The listing builds one solid part. Answer for the finished solid, in the listing's coordinates (mm). A direction names the side the tool comes from. Round coordinates to 2 decimals unless told otherwise and drop trailing zeros. Write each loop counter-clockwise with the first axis right and the second up, starting at its lowest first coordinate (ties: lowest second). Pieces come first, ordered by that corner, then holes.
Item 1: Find section B-B on x = 0. Give the vertices of the cut face in (y, z) (3 decimals), then the cut area to 3 significant figures.
Item 2: For a pull along Y with two mould halves and no side action, classify faces 1 (the face through (0.833, -2, 6)), 2 (the face through (0.2, 12.7, 11.1)), 3 (the face through (9.5, 0, 11)) as +Y half, -Y half, draft (parallel to the pull), parting line (faces both ways), or undercut.
Item 3: Find the intervals of material crossed by probe 1 along X at (y, z) = (-0.25, 9); probe 2 along X at (y, z) = (3, 5.5); probe 3 along X at (y, z) = (-2.75, 10), in increasing order.
Item 4: Find section A-A on z = 10.5. Give the vertices of the cut face in (x, y), then the cut area to 3 significant figures.
Item 5: Find section C-C on y = 8.75. Give the vertices of the cut face in (x, z) (3 decimals).
Item 6: Each of these flat-tipped pins is pushed along its axis until it touches: pin 1 (1.8 mm diameter, centred on x = -0.5, z = 9, fed in from -Y); pin 2 (2.5 mm diameter, centred on x = -2, z = 9, fed in from +Y); pin 3 (2 mm diameter, centred on y = -3, z = 3.5, fed in from -X); pin 4 (4 mm diameter, centred on x = -5.5, z = 9, fed in from -Y). Where does it stop, or does it pass through?
Item 7: A tool of negligible diameter and unlimited length cuts with its end or side. For faces 4 (the face through (1, -10, 9.525)), 5 (the face through (0, 10, 9.525)), 6 (the face through (2, -1.13, 6)), 7 (the face through (-2, 3, 12.7)), from which of +Z, -Z, +X, -X, +Y, -Y can it reach the whole face along a straight path? Write none if from no direction.
Item 8: Find section D-D on x = -6.5. Give the vertices of the cut face in (y, z) (3 decimals).
```python
from build123d import *

# Parameters (mm, degrees)
F0_R     = 9.4996
F1_DEPTH = 9.525
F2_R     = 12.7
F2_R_2   = 9.4996
F3_DEPTH = 3.175
F5_DEPTH = 25.4
F7_DEPTH = 25.4
F9_DEPTH = 25.4


with BuildPart() as f1:
    # F0 (on Top) → F1 (new body)
    with BuildSketch(Plane.XY):
        Circle(F0_R)
    extrude(amount=F1_DEPTH)

    # F2 (on face) → F3 (join)
    with BuildSketch(Plane.XY.offset(9.525)):
        Circle(F2_R)
        Circle(F2_R_2, mode=Mode.SUBTRACT)
        Circle(F2_R_2)
    extrude(amount=F3_DEPTH)

    # F4 (on face) → F5 (cut)
    with BuildSketch(Plane.XY.offset(12.7)):
        with BuildLine():
            ThreePointArc((-9.4996, 8.428974), (-12.7, 0), (-9.4996, -8.428974))
            Line((-9.4996, -8.428974), (-9.4996, 8.428974))
        make_face()
        with BuildLine():
            Line((9.4996, 8.428974), (9.4996, -8.428974))
            ThreePointArc((9.4996, -8.428974), (11.872972, -4.508053), (12.7, 0))
            ThreePointArc((12.7, 0), (11.872972, 4.508053), (9.4996, 8.428974))
        make_face()
    extrude(amount=-F5_DEPTH, mode=Mode.SUBTRACT)

    # F6 (on face) → F7 (cut)
    with BuildSketch(Plane.XY.offset(12.7)):
        with BuildLine():
            ThreePointArc((2.8575, -3.421372), (4.037881, -1.888546), (4.4577, 0))
            ThreePointArc((4.4577, 0), (4.037881, 1.888546), (2.8575, 3.421372))
            Line((2.8575, 3.421372), (2.8575, -3.421372))
        make_face()
        with BuildLine():
            Line((-2.8575, -3.421372), (-2.8575, 3.421372))
            ThreePointArc((-2.8575, 3.421372), (-4.4577, 0), (-2.8575, -3.421372))
        make_face()
    extrude(amount=-F7_DEPTH, mode=Mode.SUBTRACT)

    # F8 (on face) → F9 (cut)
    with BuildSketch(Plane(origin=(0, 0, 0), x_dir=(1, 0, 0), z_dir=(0, 0, -1))):
        Polygon((-2.8575, 2.16922), (-2.8575, -2.392801), (-0.969418, -2.392801), (-0.969418, -3.421372), (1.220574, -3.421372), (1.220574, -2.392801), (2.8575, -2.392801), (2.8575, 1.130344), (0.832597, 1.130344), (0.832597, 3.162927), (-0.79347, 3.162927), (-0.79347, 2.16922), align=None)
    extrude(amount=-F9_DEPTH, mode=Mode.SUBTRACT)


solid = f1.part
```
Check values:
1. outline: (-12.7, 9.525) - (-9.5, 9.525) - (-9.5, 0) - (-3.163, 0) - (-3.163, 12.7) - (-12.7, 12.7) - close; (3.421, 0) - (9.5, 0) - (9.5, 9.525) - (12.7, 9.525) - (12.7, 12.7) - (3.421, 12.7) - close
1. area: 178 mm2
2. face 1: undercut
2. face 2: +Y half
2. face 3: draft
3. probe 1: x = -9.5 to -4.45, 4.45 to 9.5
3. probe 2: x = -9.01 to -3.3, -2.86 to -0.97, 1.22 to 2.86, 3.3 to 9.01
3. probe 3: x = -9.5 to -3.51, -2.86 to -0.79, 0.83 to 2.86, 3.51 to 9.5
4. outline: (-9.5, -8.43) arc R12.7 ccw to (9.5, -8.43) - (9.5, 8.43) arc R12.7 ccw to (-9.5, 8.43) - close; hole (-2.86, -3.42) - (-2.86, -2.17) - (-0.79, -2.17) - (-0.79, -3.16) - (0.83, -3.16) - (0.83, -1.13) - (2.86, -1.13) - (2.86, -3.42) arc R4.46 ccw to (4.46, 0) arc R4.46 ccw to (2.86, 3.42) - (2.86, 2.39) - (1.22, 2.39) - (1.22, 3.42) - (-0.97, 3.42) - (-0.97, 2.39) - (-2.86, 2.39) - (-2.86, 3.42) arc R4.46 ccw to start
4. area: 390 mm2
5. outline: (-9.205, 9.525) - (-3.699, 9.525) - (-3.699, 0) - (3.699, 0) - (3.699, 9.525) - (9.205, 9.525) - (9.205, 12.7) - (-9.205, 12.7) - close
6. pin 1: stops at y = -12.7
6. pin 2: stops at y = 12.67
6. pin 3: stops at x = -9.29
6. pin 4: stops at y = -12.19
7. face 4: -Z, -Y
7. face 5: -Z, +Y
7. face 6: +Z, -Z
7. face 7: +Z, +X, -X, +Y, -Y
8. outline: (-10.911, 9.525) - (-6.928, 9.525) - (-6.928, 0) - (6.928, 0) - (6.928, 9.525) - (10.911, 9.525) - (10.911, 12.7) - (-10.911, 12.7) - close
